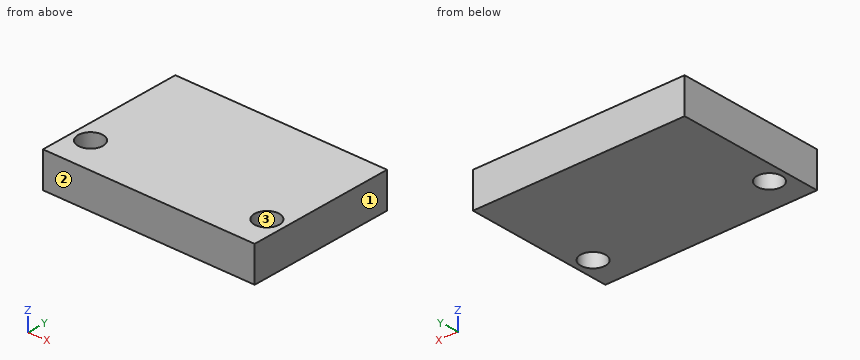
Autodesk Inventor part; units mm, degrees
ref_plane "YZ Plane" through (0, 0, 0) normal (1, 0, 0) x (0, 1, 0)
ref_plane "XZ Plane" through (0, 0, 0) normal (0, 1, 0) x (-1, 0, 0)
ref_plane "XY Plane" through (0, 0, 0) normal (0, 0, 1) x (1, 0, 0)
sketch "Boceto1" plane through (0, 0, 0) normal (0, 0, 1) x (1, 0, 0)
  line L0 (-12.441, 14.2571) -> (17.559, 14.2571)
  line L1 (17.559, 14.2571) -> (17.559, -15.7429)
  line L2 (17.559, -15.7429) -> (-12.441, -15.7429)
  line L3 (-12.441, -15.7429) -> (-12.441, 14.2571)
  point P0 (0, 0)
  dimension "d0" = 30
extrude "Extrusión1" add sketch "Boceto1" along normal blind 5
sketch "Boceto2" plane through (0, 0, 5) normal (0, 0, 1) x (1, 0, 0)
  line L0 (17.559, 14.2571) -> (17.559, -15.7429)
  line L1 (-12.441, 14.2571) -> (17.559, 14.2571)
  line L2 (-12.441, -15.7429) -> (-12.441, 14.2571)
  circle A0 centre (-9.941, -1.9929) radius 1.75
  circle A1 centre (15.059, -1.9929) radius 1.75
  point P0 (0, 0)
  dimension "d3" = 2.5
  dimension "d4" = 2.5
  dimension "d5" = 16.25
  dimension "d6" = 16.25
extrude "Extrusión2" cut sketch "Boceto2" against normal blind 5
move faces "Desplazar cara1" translate (0, 3, 0) faces at (7.559, -15.7429, 1.6667)
move faces "Desplazar cara2" translate (0, 5, 0) faces at (7.559, -12.7429, 1.6667)
move faces "Desplazar cara3" translate (0, 1, 0) faces at (7.559, -7.7429, 1.6667)
properties part number "tapa polea x 2"
Verification items for the finished model (mm, model axes). Face numbers are marked on the shaded views. Coordinates: 2 decimals unless noted, no trailing zeros. Write each loop counter-clockwise with the first axis right and the second up, starting at its lowest first coordinate (ties: lowest second). Pieces come first, ordered by that corner, then holes. Notation, with made-up numbers: M 18.25,-7.75 L 46.25,-7.75 A20 ccw 46.25,26.25 Z; hole C 51,3.5 d4. An arc over 180 degrees is marked long. Answer as a JSON object with one key per item and string values. Group by question number.
(1) Cross-section at A-A, the plane x = -10.5. Record the cut outline in (y, z), and give its area (3 significant figures).
(2) Gauge pin test, flat end, axial feed: pin 1 (3 mm diameter, centred on x = -9.94, y = -1.99, fed in from -Z). Record the tip position at first contact, or that the pin passes through.
(3) Release check for a two-part mould opening along X. For the marked faces 1, 2 and 3 record: +X half, -X half, draft (parallel to the pull), parting line (faces both ways), or undercut.
(4) Material ranges on line 1 (Y direction, x = -10, z = 2.1); line 2 (Y direction, x = 14.75, z = 4.6); line 3 (X direction, y = -2.25, z = 1.1), recorded low to high.
(5) Cross-section at C-C, the plane z = 4.35. Record the cut outline in (x, y), and give its area (3 significant figures).
(6) Cross-section at B-B, the plane y = -3. Record the cut outline in (x, z), and give its area (3 significant figures).
Reply:
{
 "1": {"outline": "M -6.74,0 L -3.65,0 L -3.65,5 L -6.74,5 Z; M -0.33,0 L 14.26,0 L 14.26,5 L -0.33,5 Z", "area": "88.4 mm²"},
 "2": {"pin 1": "through"},
 "3": {"face 1": "+X half", "face 2": "draft", "face 3": "undercut"},
 "4": {"line 1": "-6.74 to -3.74, -0.24 to 14.26", "line 2": "-6.74 to -3.72, -0.27 to 14.26", "line 3": "-12.44 to -11.67, -8.21 to 13.33, 16.79 to 17.56"},
 "5": {"outline": "M -12.44,-6.74 L 17.56,-6.74 L 17.56,14.26 L -12.44,14.26 Z; hole C -9.94,-1.99 d3.5; hole C 15.06,-1.99 d3.5", "area": "611 mm²"},
 "6": {"outline": "M -12.44,0 L -11.37,0 L -11.37,5 L -12.44,5 Z; M -8.51,0 L 13.63,0 L 13.63,5 L -8.51,5 Z; M 16.49,0 L 17.56,0 L 17.56,5 L 16.49,5 Z", "area": "121 mm²"}
}
